Verification items for the finished model (mm, model axes). A direction names the side the tool comes from. Round coordinates to 2 decimals unless told otherwise and drop trailing zeros. Order: outer loops, then holes, each group sorted by start corner. A loop starts at its lowest first (then second) coordinate and runs counter-clockwise, first axis right, second up. Notation, with made-up numbers: (-37.5, 22.5) -> (-11.5, 22.5) arc R20 cw to (-11.5, 57.5) -> close; hole circle Ø11 at (-22.75, 50.5). An arc over 180 degrees is marked (long way). Put each result on its own line as item: value.
from build123d import *

# Parameters (mm, degrees)
F1_DEPTH = 146
F4_W     = 216
F4_H     = 216
F2_W     = 210
F2_H     = 210
F6_W     = 200
F6_H     = 200
F7_DEPTH = 12
F8_W     = 45
F8_H     = 25
F9_DEPTH = 180


with BuildPart() as f1:
    # F0 (on Top) → F1 (new body)
    with BuildSketch(Plane.XY):
        Polygon((25, 0), (0, 0), (0, -25), (5, -25), (5, -5), (25, -5), align=None)
    extrude(amount=F1_DEPTH)



with BuildPart() as f1b:
    # F0 (on Top) → F1, piece 2 (new body)
    with BuildSketch(Plane.XY):
        Polygon((210, 0), (185, 0), (185, -5), (205, -5), (205, -25), (210, -25), align=None)
    extrude(amount=F1_DEPTH)


with BuildPart() as f1c:
    # F0 (on Top) → F1, piece 3 (new body)
    with BuildSketch(Plane.XY):
        Polygon((5, -185), (0, -185), (0, -210), (25, -210), (25, -205), (5, -205), align=None)
    extrude(amount=F1_DEPTH)


with BuildPart() as f1d:
    # F0 (on Top) → F1, piece 4 (new body)
    with BuildSketch(Plane.XY):
        Polygon((185, -210), (210, -210), (210, -185), (205, -185), (205, -205), (185, -205), align=None)
    extrude(amount=F1_DEPTH)


with BuildPart() as f1_1:
    add(f1.part)

    add(f1b.part)  # F5 merges F1b

    add(f1c.part)  # F5 merges F1c

    add(f1d.part)  # F5 merges F1d
    # F4 (on offset) → F5 section 0
    with BuildSketch(Plane.XY.offset(158)):
        with Locations((105, -105)):
            Rectangle(F4_W, F4_H)
    # F2 (on face) → F5 section 1
    with BuildSketch(Plane.XY.offset(146)):
        with Locations((105, -105)):
            Rectangle(F2_W, F2_H)
    loft()

    # F6 (on face) → F7 (cut)
    with BuildSketch(Plane.XY.offset(158)):
        with Locations((105, -105)):
            Rectangle(F6_W, F6_H)
    extrude(amount=-F7_DEPTH, mode=Mode.SUBTRACT)

    # F8 (on Top) → F9 (cut)
    with BuildSketch(Plane.XY):
        with Locations((70, 7.5)):
            Rectangle(F8_W, F8_H)
    extrude(amount=F9_DEPTH, mode=Mode.SUBTRACT)


solid = f1_1.part
Item 1: Material ranges on L1, parallel to Y at x = 20.5, z = 77; L2, parallel to X at y = -41.5, z = 151.5 (3 decimals); L3, parallel to X at y = -83.5, z = 148, recorded low to high. Write a range as [from, to].
Check sheet entries:
L1: y = [-210, -205], [-5, 0]
L2: x = [-1.375, 5], [205, 211.375]
L3: x = [-0.5, 5], [205, 210.5]
Item 2: Gauge pin test, flat ends, axial feed: pin 1 Ø4 at (x, y) = (3, -100.5) entering from -Z; pin 2 Ø5.5 at (y, z) = (-1.5, 45.5) entering from -X; pin 3 Ø4 at (y, z) = (-2.5, 89.5) entering from +X. Record the tip position at first contact, or that the pin passes through.
Check sheet entries:
pin 1: stops at z = 146
pin 2: stops at x = 0
pin 3: stops at x = 210
Item 3: Tool access check on faces 1 (the flat face through (5, -128, 150)), 2 (the flat face through (197, -210, 72)), 3 (the flat face through (47.5, -2, 152)), 4 (the flat face through (0, -197, 72)). Record the directions out of +Z, -Z, +X, -X, +Y, -Y that give a thin tool (end or side, any length) a straight path to the whole face; none if there is none.
Check sheet entries:
face 1: +Z, -Z
face 2: -Z, +X, -X, -Y
face 3: +Z, -Z, +Y
face 4: -Z, -X, +Y, -Y
Item 4: Release check for a two-part mould opening along Y. For faces 5 (the flat face through (12, -210, 72)), 6 (the flat face through (205, -128, 150)), 7 (the flat face through (0, -12, 72)), 8 (the flat face through (13, 0, 72)) record: +Y half, -Y half, draft (parallel to the pull), parting line (faces both ways), or undercut.
Check sheet entries:
face 5: -Y half
face 6: undercut
face 7: draft
face 8: +Y half
Item 5: Section check A-A on z = 105.5. Record the boundary of the cut face in (x, y), then the cut area to 3 significant figures.
Check sheet entries:
outline: (0, -210) -> (25, -210) -> (25, -205) -> (5, -205) -> (5, -185) -> (0, -185) -> close; (0, -25) -> (5, -25) -> (5, -5) -> (25, -5) -> (25, 0) -> (0, 0) -> close; (185, -210) -> (210, -210) -> (210, -185) -> (205, -185) -> (205, -205) -> (185, -205) -> close; (185, -5) -> (205, -5) -> (205, -25) -> (210, -25) -> (210, 0) -> (185, 0) -> close
area: 900 mm^2
